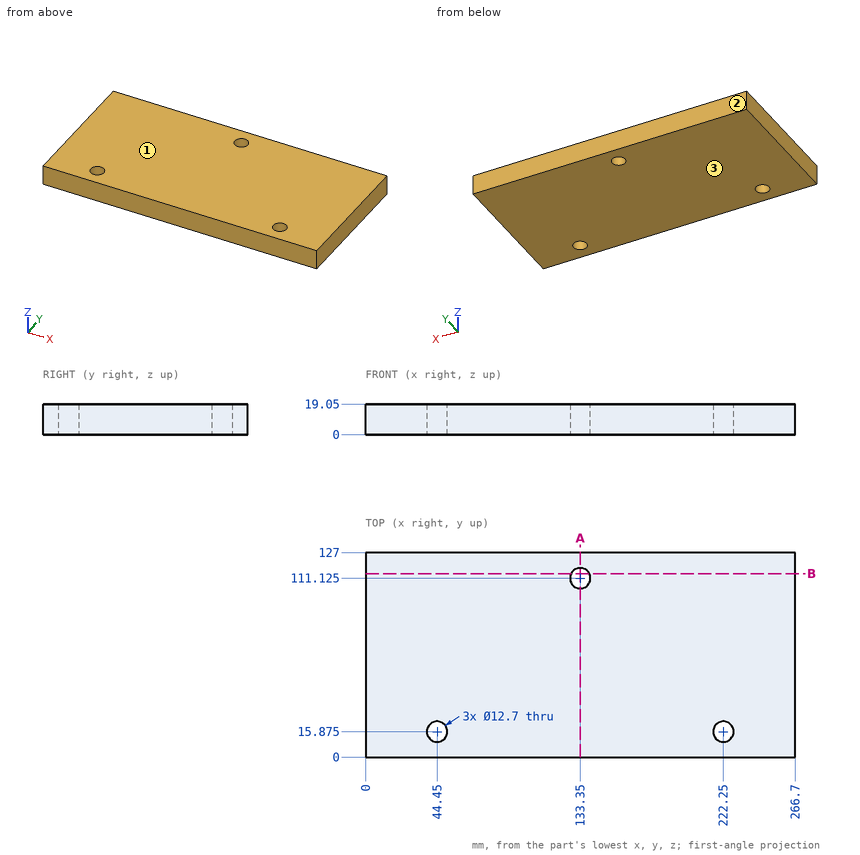
Print and shaded views of the part. All mm, measured from the part's lowest x, y and z. Coordinates: 2 decimals unless noted, no trailing zeros. Loops run counter-clockwise (first coordinate to the right, second up) from the corner with the lowest first, then second, coordinate; pieces in that order, holes last. Notation, with made-up numbers: (47, 70) - (68, 70) arc R28 cw to (68, 91) - close; hole circle Ø2 at (-18.75, 17). An arc over 180 degrees is marked (long way). Write item = value, one per line. Start each with the question number.
Item 1: Mould opens along Z. For the marked faces 1, 2 and 3 say: released by +Z, released by -Z, zero draft, split by the parting line, or undercut.
Item 2: Wall check: L1, parallel to X at y = 14, z = 9.5; L2, parallel to Y at x = 44.45, z = 5.75 (3 decimals); L3, parallel to X at y = 18.5, z = 7.75. Give the ranges that are in metal, low to high. Write a range as from..to.
Item 3: Cut at A-A, the plane x = 133.35. Give the cut face in (y, z) (3 decimals).
Item 4: Flat gauge pin, fed straight in: pin 1 Ø11.5 at (x, y) = (44.45, 15.875) entering from +Z. Where does the tip first touch, or does it go through?
Item 5: Cut at B-B, the plane y = 114. Give the cut face in (x, z).
The answers:
q1.face_1 = released by +Z
q1.face_2 = zero draft
q1.face_3 = released by -Z
q2.L1 = 0..38.38, 50.52..216.18, 228.32..266.7
q2.L2 = 0..9.525, 22.225..127
q2.L3 = 0..38.67, 50.23..216.47, 228.03..266.7
q3.outline = (0, 0) - (104.775, 0) - (104.775, 19.05) - (0, 19.05) - close; (117.475, 0) - (127, 0) - (127, 19.05) - (117.475, 19.05) - close
q4.pin_1 = through
q5.outline = (0, 0) - (127.69, 0) - (127.69, 19.05) - (0, 19.05) - close; (139.01, 0) - (266.7, 0) - (266.7, 19.05) - (139.01, 19.05) - close
